Job drawing, mm, ordinate dimensions from the low corner. One solid piece. Coordinates: 2 decimals unless noted, no trailing zeros. Order: outer loops, then holes, each group sorted by start corner. A loop starts at its lowest first (then second) coordinate and runs counter-clockwise, first axis right, second up. Notation, with made-up numbers: M 60.5,14 L 95.5,14 A18 cw 95.5,23 Z; hole C 32,-25.5 d7. An arc over 180 degrees is marked long. Write item = value, one per line.
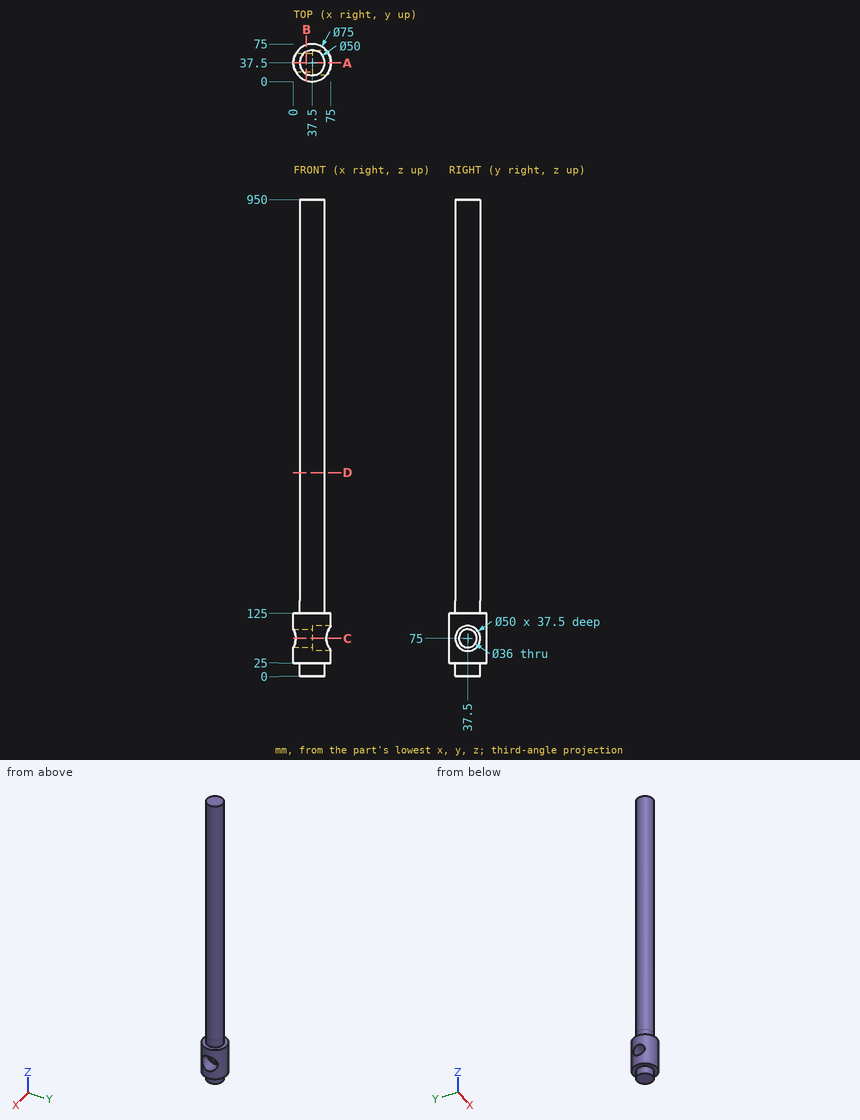
(1) Wall check: line 1 (Z direction, x = 60.5, y = 37.5); line 2 (Z direction, x = 70, y = 39); line 3 (Z direction, x = 14.5, y = 15). Give the ranges that are in metal, low to high. Write a range as from..to.
Evaluation:
line_1 = 0..50, 100..950
line_2 = 25..50.05, 99.95..125
line_3 = 25..125
(2) Slice it at D-D, the plane z = 405.5. Write the cut outline in (x, y).
Evaluation:
outline = C 37.5,37.5 d50
(3) Slice it at A-A, the plane y = 37.5. Write the cut outline in (x, z), then the cut area to 3 significant figures.
Evaluation:
outline = M 0,25 L 12.5,25 L 12.5,0 L 62.5,0 L 62.5,25 L 75,25 L 75,50 L 37.5,50 L 37.5,57 L 0,57 Z; M 0,93 L 37.5,93 L 37.5,100 L 75,100 L 75,125 L 62.5,125 L 62.5,950 L 12.5,950 L 12.5,125 L 0,125 Z
area = 46,800 mm²
(4) Pin check, flat tips, straight feed: pin 1 Ø12 at (y, z) = (14, 503.5) entering from -X; pin 2 Ø2 at (x, z) = (58.5, 458) entering from -Y; pin 3 Ø1 at (y, z) = (58, 327.5) entering from -X. Stop position of each tip, or through.
Evaluation:
pin_1 = 19.65
pin_2 = 22.5
pin_3 = 22.5
(5) Slice it at B-B, the plane x = 26. Write the cut outline in (y, z), then the cut area to 3 significant figures.
Evaluation:
outline = M 1.81,25 L 15.3,25 L 15.3,0 L 59.7,0 L 59.7,25 L 73.19,25 L 73.19,125 L 59.7,125 L 59.7,950 L 15.3,950 L 15.3,125 L 1.81,125 Z; hole C 37.5,75 d36
area = 43,900 mm²
(6) Slice it at C-C, the plane z = 75. Write the cut outline in (x, y), then the cut area to 3 significant figures.
Evaluation:
outline = M 4.6,19.5 A37.5 ccw 65.45,12.5 L 37.5,12.5 L 37.5,19.5 Z; M 4.6,55.5 L 37.5,55.5 L 37.5,62.5 L 65.45,62.5 A37.5 ccw Z
area = 1,400 mm²
